For this review, use the dimensioned drawing (mm, ordinates from the lowest corner) and the shaded views. Give positions to 0.01 mm unless a question says otherwise; leave off trailing zeros. Order: outer loops, then holes, each group sorted by start corner. A loop starts at its lowest first (then second) coordinate and runs counter-clockwise, first axis right, second up. Notation, with made-up numbers: (9, -37.75) -> (57, -37.75) arc R24 cw to (57, -12.75) -> close; hole circle Ø5 at (17.25, 22). An arc over 180 degrees is marked (long way). One line per item, written item: value. Start each with the question number.
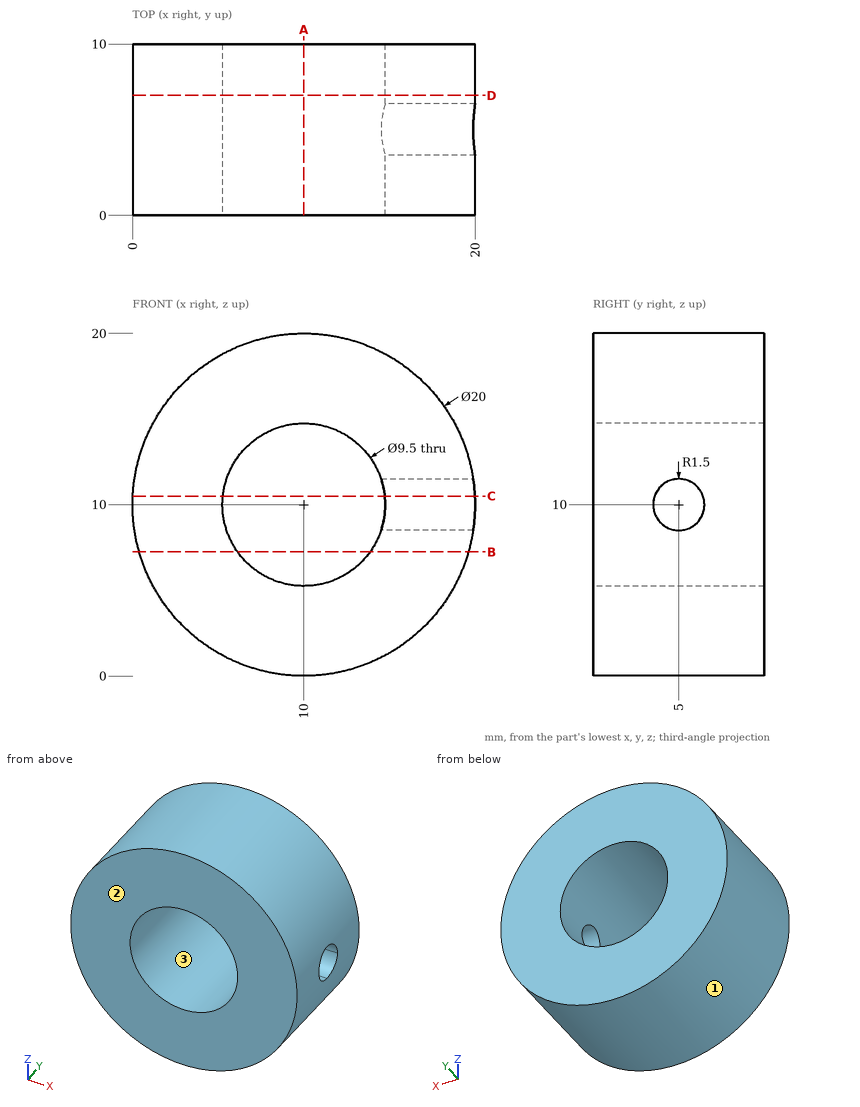
Q1. For line 1 along Z through (x, y) = (10, 5.25); line 2 along Z through (x, y) = (11.5, 9); line 3 along Y through (x, z) = (15, 10.75), list the stretches that pass through material, from the lowest coordinate up.
Q2. Mouldability with a two-part tool opening along Z and no side actions: class the marked faces 1, 2 and 3 as pulls with the +Z half, pulls with the -Z half, needs draft (parallel to the pull), parting line crosses it, or undercut.
Q3. For pin 1 Ø2 at (x, y) = (13.5, 5) entering from +Z; pin 2 Ø3 at (y, z) = (5, 9.5) entering from -X; pin 3 Ø2 at (x, y) = (14.5, 7.5) entering from -Z; pin 4 Ø2 at (x, y) = (12.5, 7) entering from +Z, all flat-tipped, find the tip position at first contact; note any pin that passes through.
Q4. Take a section at B-B (z = 7.25). State the section outline as (x, y) points, and give its area (3 significant figures).
Q5. Take a section at D-D (y = 7). State the section outline as (x, z) points, and give its area (3 significant figures).
Q6. Take a section at A-A (x = 10). State the section outline as (y, z) points.
Q7. Take a section at C-C (z = 10.5). State the section outline as (x, y) points.
Answers below:
1. line 1: z = 0 to 5.25, 14.75 to 20
1. line 2: z = 0.11 to 5.49, 14.51 to 19.89
1. line 3: y = 0 to 3.7, 6.3 to 10
2. face 1: parting line crosses it
2. face 2: needs draft
2. face 3: undercut
3. pin 1: stops at z = 19.68
3. pin 2: stops at x = 0
3. pin 3: stops at z = 0.63
3. pin 4: stops at z = 19.89
4. outline: (0.39, 0) -> (6.13, 0) -> (6.13, 10) -> (0.39, 10) -> close; (13.87, 0) -> (19.61, 0) -> (19.61, 10) -> (13.87, 10) -> close
4. area: 115 mm²
5. outline: circle Ø20 at (10, 10); hole circle Ø9.5 at (10, 10)
5. area: 243 mm²
6. outline: (0, 0) -> (10, 0) -> (10, 5.25) -> (0, 5.25) -> close; (0, 14.75) -> (10, 14.75) -> (10, 20) -> (0, 20) -> close
7. outline: (0.01, 0) -> (5.28, 0) -> (5.28, 10) -> (0.01, 10) -> close; (14.72, 0) -> (19.99, 0) -> (19.99, 3.59) -> (14.72, 3.59) -> close; (14.72, 6.41) -> (19.99, 6.41) -> (19.99, 10) -> (14.72, 10) -> close
